```python
from build123d import *

# Parameters (mm, degrees)
F0_R     = 19.05
F1_DEPTH = 9.525
F2_R     = 5.08
F3_R     = 1.731017
F4_DEPTH = 19.05


with BuildPart() as f1:
    # F0 (on Front) → F1 (new body, symmetric)
    with BuildSketch(Plane.XZ):
        Circle(F0_R)
    extrude(amount=F1_DEPTH, both=True)

    # F2
    f2_edges = [f1.edges().sort_by_distance(p)[0] for p in [
        (-19.05, -9.525, 0),
        (-19.05, 9.525, 0),
    ]]
    fillet(f2_edges, radius=F2_R)

    # F3 (on face) → F4 (cut)
    with BuildSketch(Plane.XZ.offset(9.525)):
        Circle(F3_R)
    extrude(amount=-F4_DEPTH, mode=Mode.SUBTRACT)


solid = f1.part
```
Verification items for the finished model (mm, model axes). Round coordinates to 2 decimals unless told otherwise and drop trailing zeros. Order: outer loops, then holes, each group sorted by start corner. A loop starts at its lowest first (then second) coordinate and runs counter-clockwise, first axis right, second up. Notation, with made-up numbers: (14.5, -21.75) - (53.5, -21.75) arc R28 cw to (53.5, -1.75) - close; hole circle Ø3 at (-30.5, 41). An arc over 180 degrees is marked (long way). Use CSV: the item, a comma, the result in double quotes.
(1) Thickness scan on probe 1 along Z at (x, y) = (0, -2.75); probe 2 along Z at (x, y) = (4.5, 6.25); probe 3 along X at (y, z) = (-4.5, 1). Record the ranges inside material, lowest first. Write a range as from..to.
Entries:
probe 1,"-19.05..-1.73, 1.73..19.05"
probe 2,"-18.17..18.17"
probe 3,"-19.02..-1.41, 1.41..19.02"
(2) Section check A-A on z = 0. Record the boundary of the cut face in (x, y) (3 decimals), and give its area (3 significant figures).
Entries:
outline,"(-19.05, -4.445) arc R5.08 ccw to (-13.97, -9.525) - (-1.731, -9.525) - (-1.731, 9.525) - (-13.97, 9.525) arc R5.08 ccw to (-19.05, 4.445) - close; (1.731, -9.525) - (13.97, -9.525) arc R5.08 ccw to (19.05, -4.445) - (19.05, 4.445) arc R5.08 ccw to (13.97, 9.525) - (1.731, 9.525) - close"
area,"638 mm^2"
(3) Gauge pin test, flat ends, axial feed: pin 1 Ø1.5 at (y, z) = (-4, 4) entering from -X; pin 2 Ø10 at (x, y) = (-6, -3) entering from +Z; pin 3 Ø6 at (y, z) = (0.5, -12.5) entering from +X. Record the tip position at first contact, or that the pin passes through.
Entries:
pin 1,"x = -18.77"
pin 2,"z = 19.02"
pin 3,"x = 16.51"
(4) Section check D-D on y = 5. Record the boundary of the cut face in (x, z), and give its area (3 significant figures).
Entries:
outline,"circle Ø38.04 at (0, 0); hole circle Ø3.46 at (0, 0)"
area,"1,130 mm^2"
(5) Section check C-C on y = 1.5. Record the boundary of the cut face in (x, z).
Entries:
outline,"circle Ø38.1 at (0, 0); hole circle Ø3.46 at (0, 0)"
(6) Section check B-B on x = 0. Record the boundary of the cut face in (y, z) (3 decimals).
Entries:
outline,"(-9.525, -13.97) arc R5.08 ccw to (-4.445, -19.05) - (4.445, -19.05) arc R5.08 ccw to (9.525, -13.97) - (9.525, -1.731) - (-9.525, -1.731) - close; (-9.525, 1.731) - (9.525, 1.731) - (9.525, 13.97) arc R5.08 ccw to (4.445, 19.05) - (-4.445, 19.05) arc R5.08 ccw to (-9.525, 13.97) - close"
(7) Mould release check, pull along X, two halves, no side actions. Record for faces 1 (the face through (-15.12, -0.06, -11.59)), 2 (the face through (-0.38, -0.13, -1.69)), 3 (the face through (3, 9.525, 0)): released by +X, released by -X, zero draft, split by the parting line, or undercut.
Entries:
face 1,"split by the parting line"
face 2,"undercut"
face 3,"zero draft"
